Build history of the part. All positions in model axes, mm. A direction names the side the tool comes from. Round coordinates to 2 decimals unless told otherwise and drop trailing zeros. Write each loop counter-clockwise with the first axis right and the second up, starting at its lowest first coordinate (ties: lowest second). Pieces come first, ordered by that corner, then holes. Notation, with made-up numbers: (82.5, 3.25) -> (112.5, 3.25) arc R6 ccw to (112.5, 13.25) -> close; hole circle Ø2 at (17, 23). An arc over 180 degrees is marked (long way). One line per question, with ' | ' between items.
from build123d import *

# Parameters (mm, degrees)
SKETCH_1_R      = 39
EXTRUDE_1_DEPTH = 34
CHAMFER_1_SIZE  = 5
CHAMFER_2_SIZE  = 0.5


with BuildPart() as part:
    # Эскиз1 → Бобышка-Вытянуть1 (new, symmetric)
    with BuildSketch(Plane(origin=(0, 0, 0), x_dir=(0, 0, -1), z_dir=(1, 0, 0))):
        Circle(SKETCH_1_R)
        with BuildLine():
            Line((-7, 26.3), (7, 26.3))
            Line((7, 26.3), (7, 21.38340478))
            ThreePointArc((7, 21.38340478), (0, -22.5), (-7, 21.38340478))
            Line((-7, 21.38340478), (-7, 26.3))
        make_face(mode=Mode.SUBTRACT)
    extrude(amount=EXTRUDE_1_DEPTH, both=True)

    # Фаска1
    chamfer_1_edges = [part.edges().sort_by_distance(p)[0] for p in [
        (-34, 0, 39),
    ]]
    chamfer(chamfer_1_edges, length=CHAMFER_1_SIZE)

    # Фаска2
    chamfer_2_edges = [part.edges().sort_by_distance(p)[0] for p in [
        (34, 26.3, 0),
        (34, 23.84170239, 7),
        (-34, -22.5, 0),
        (-34, 23.84170239, -7),
        (-34, 26.3, 0),
        (-34, 23.84170239, 7),
        (34, -22.5, 0),
        (34, 23.84170239, -7),
    ]]
    chamfer(chamfer_2_edges, length=CHAMFER_2_SIZE)

    # Эскиз2 → Вырез-Повернуть1 (revolve, cut)
    with BuildSketch(Plane.XY, mode=Mode.PRIVATE) as cut_revolve_1_sk:
        Polygon((34, 35), (29, 35), (29, 37), (27, 39), (34, 39), align=None)
    revolve(cut_revolve_1_sk.sketch.rotate(Axis((0, 0, 0), (1, 0, 0)), 90), axis=Axis((0, 0, 0), (1, 0, 0)), mode=Mode.SUBTRACT)


solid = part.part
(1) Slice it at B-B (y = 0). Write the cut outline in (x, z), then the cut area to 3 significant figures.
Calculated:
outline: (-34, -34) -> (-29, -39) -> (27, -39) -> (29, -37) -> (29, -35) -> (34, -35) -> (34, -23) -> (33.5, -22.5) -> (-33.5, -22.5) -> (-34, -23) -> close; (-34, 23) -> (-33.5, 22.5) -> (33.5, 22.5) -> (34, 23) -> (34, 35) -> (29, 35) -> (29, 37) -> (27, 39) -> (-29, 39) -> (-34, 34) -> close | area: 2,170 mm2
(2) Wall check: line 1 (Y direction, x = -5, z = 0); line 2 (Y direction, x = -24.5, z = 5); line 3 (Z direction, x = -31, y = -1). Give the ranges that are in metal, low to high. Write a range as from..to.
Calculated:
line 1: -39..-22.5, 26.3..39 | line 2: -38.68..-21.94, 26.3..38.68 | line 3: -36.99..-22.48, 22.48..36.99
(3) 3-axis set-ups, long thin cutter, end or side, ignore diameter. For faces 4 (the flat face through (0, 24, -7)), 5 (the flat face through (29, 33, -14)), 6 (the flat face through (-34, -22.2, -7.1)): which of +Z, -Z, +X, -X, +Y, -Y reach the whole face in a straight line?
Calculated:
face 4: +X, -X | face 5: +X | face 6: +Z, -Z, -X, +Y, -Y
(4) Drop flat-ended pins along their axis: pin 1 (5.5 mm diameter, centred on x = -4.5, y = 24.5, fed in from +Z); pin 2 (10 mm diameter, centred on x = -17.5, z = 17.5, fed in from -Y); pin 3 (3 mm diameter, centred on x = -1.5, z = -22.5, fed in from -Y). Give the stop position or say it passes through.
Calculated:
pin 1: z = 32.37 | pin 2: y = -36.94 | pin 3: y = -32.86
(5) Mould opens along Z. For faces 1 (the flat face through (0, 24, 7)), 2 (the flat face through (34, -23, -7)), 3 (the conical face through (28.875, 36.242, -8.048)) say: pulls with the +Z half, pulls with the -Z half, needs draft (parallel to the pull), parting line crosses it, or undercut.
Calculated:
face 1: undercut | face 2: needs draft | face 3: parting line crosses it
(6) Slice it at A-A (z = 0). Write the cut outline in (x, y), then the cut area to 3 significant figures.
Calculated:
outline: (-34, -34) -> (-29, -39) -> (27, -39) -> (29, -37) -> (29, -35) -> (34, -35) -> (34, -23) -> (33.5, -22.5) -> (-33.5, -22.5) -> (-34, -23) -> close; (-34, 26.8) -> (-33.5, 26.3) -> (33.5, 26.3) -> (34, 26.8) -> (34, 35) -> (29, 35) -> (29, 37) -> (27, 39) -> (-29, 39) -> (-34, 34) -> close | area: 1,920 mm2
(7) Slice it at C-C (x = 25). Write the cut outline in (y, z).
Calculated:
outline: circle Ø78 at (0, 0); hole (21.38, -7) -> (26.3, -7) -> (26.3, 7) -> (21.38, 7) arc R22.5 ccw (long way) to start
